Autodesk Inventor part; units mm, degrees
ref_plane "Work Plane1" through (-27.5, -47.498, -12.7) normal (0, 0, 1) x (1, 0, 0)
ref_plane "Work Plane2" through (-27.5, -47.498, -20.1034) normal (0, -1, 0) x (1, 0, 0)
ref_plane "YZ Plane" through (0, 0, 0) normal (1, 0, 0) x (0, 1, 0)
sketch "Sketch1" plane through (0, 0, 0) normal (0, 0, 1) x (1, 0, 0)
  line L0 (4.2148, -12.63) -> (4.2148, -18.63)
  line L1 (0.6968, -12.63) -> (4.2148, -12.63)
  line L2 (0.6968, 12.63) -> (0.6968, -12.63)
  line L3 (16.6988, 12.63) -> (0.6968, 12.63)
  line L4 (16.6988, 17.202) -> (16.6988, 12.63)
  line L5 (21.6388, 17.202) -> (16.6988, 17.202)
  line L6 (21.6388, 12.63) -> (21.6388, 17.202)
  line L7 (23.7568, 12.63) -> (21.6388, 12.63)
  line L8 (23.7568, 18.63) -> (23.7568, 12.63)
  line L9 (-23.7568, 18.63) -> (23.7568, 18.63)
  line L10 (-23.7568, 12.63) -> (-23.7568, 18.63)
  line L11 (-21.6388, 12.63) -> (-23.7568, 12.63)
  line L12 (-21.6388, 17.202) -> (-21.6388, 12.63)
  line L13 (-16.6988, 17.202) -> (-21.6388, 17.202)
  line L14 (-16.6988, 12.63) -> (-16.6988, 17.202)
  line L15 (-0.6968, 12.63) -> (-16.6988, 12.63)
  line L16 (-0.6968, -12.63) -> (-0.6968, 12.63)
  line L17 (-4.2148, -12.63) -> (-0.6968, -12.63)
  line L18 (-4.2148, -18.63) -> (-4.2148, -12.63)
  line L19 (4.2148, -18.63) -> (-4.2148, -18.63)
  line L20 (0, 12.63) -> (10, 12.63)
  line L21 (10, 12.63) -> (-10, 12.63)
  line L22 (10, 12.63) -> (10, -22.37)
  line L23 (10, -22.37) -> (-10, -22.37)
  line L24 (-10, -22.37) -> (-10, 12.63)
  line L25 (-10, 12.63) -> (10, 12.63)
  line L26 (10, 12.63) -> (10, -22.37)
  point P0 (0, 0)
  dimension "d0" = 10
  dimension "d1" = 20
  dimension "d2" = 35
extrude "Extrusion1" add sketch "Sketch1" along normal blind 2 contours L1 L2 L3 L22 L23 L24 L15 L16 L17 L18 L19 L0 | L0 L19 L18 L17 L16 L21 L20 L2 L1
sketch "Sketch2" plane through (0, 0, 0) normal (0, 0, -1) x (-1, 0, 0)
  line L0 (9.2308, -18.63) -> (23.7568, -18.63)
  line L1 (4.2148, -19.63) -> (-4.2148, -19.63)
  line L2 (10, 12.63) -> (10, -22.37)
  line L3 (-10, -22.37) -> (-10, 12.63)
  line L4 (10, -19.63) -> (-10, -19.63)
  line L5 (-10, -19.63) -> (-10, -22.37)
  line L6 (-10, -22.37) -> (10, -22.37)
  line L7 (10, -22.37) -> (10, -19.63)
  point P0 (0, 0)
ref_plane "Work Plane1" through (-27.5, -47.498, -12.7) normal (0, 0, 1) x (1, 0, 0)
extrude "Extrusion2" add sketch "Sketch2" along normal up to surface (12.7 mm away)
sketch "Sketch3" plane through (-10, -22.37, 2) normal (0, -1, 0) x (1, 0, 0)
  line L0 (0, -14.7) -> (0, 0)
  line L1 (0, -14.7) -> (0, -12.7)
  line L2 (20, -14.7) -> (20, 0)
  line L3 (0, -12.7) -> (20, -12.7)
  line L4 (20, -12.7) -> (20, -14.7)
  line L5 (20, -14.7) -> (0, -14.7)
  line L6 (0, -14.7) -> (0, -12.7)
  point P0 (10, -2)
  dimension "d7" = 2
ref_plane "Work Plane2" through (-27.5, -47.498, -20.1034) normal (0, -1, 0) x (1, 0, 0)
extrude "Extrusion3" add sketch "Sketch3" along normal up to surface (25.128 mm away)
properties part number "SyringeConnector"
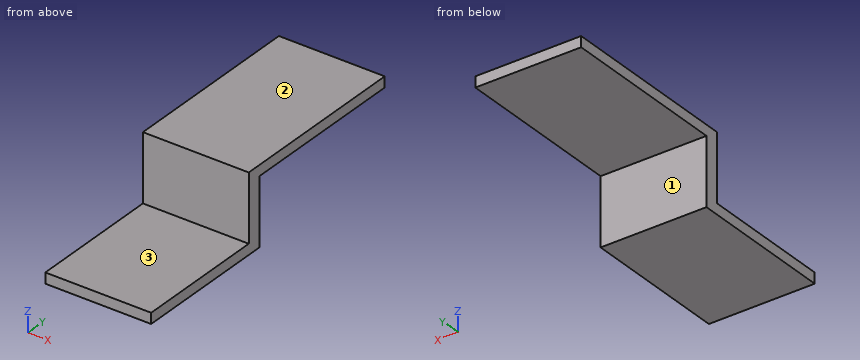
Build history of the part. All positions in model axes, mm. Face numbers are marked on the shaded views. A direction names the side the tool comes from. Coordinates: 2 decimals unless noted, no trailing zeros. Write each loop counter-clockwise with the first axis right and the second up, starting at its lowest first coordinate (ties: lowest second). Pieces come first, ordered by that corner, then holes.
(1) Drill centre lines: line 1 (Y direction, x = 9.25, z = -1.5); line 2 (Z direction, x = -5.75, y = -9.5); line 3 (Z direction, x = -4, y = -30.5). Where is each one in solid material? Low to high.
(2) Cut at C-C on y = -29. List the corners of the cut face in (x, z), and give its area (3 significant figures).
(3) Cut at B-B on z = -2. List the corners of the cut face in (x, y).
(4) 3-axis set-ups, long thin cutter, end or side, ignore diameter. For the marked faces 1, 2 and 3: which of +Z, -Z, +X, -X, +Y, -Y reach the whole face in a straight line?
(5) Cut at A-A on x = -6.5. List the corners of the cut face in (y, z).
(6) Pin check, flat tips, straight feed: pin 1 Ø3 at (x, z) = (-4, -9) entering from +Y; pin 2 Ø10 at (x, y) = (3, -8.5) entering from -Z. Stop position of each tip, or through.
Working result:
1. line 1: y = -22.37 to -19.63
1. line 2: z = 0 to 2
1. line 3: z = -12.7 to -10.7
2. outline: (-10, -12.7) - (10, -12.7) - (10, -10.7) - (-10, -10.7) - close
2. area: 40.0 mm2
3. outline: (-10, -22.37) - (10, -22.37) - (10, -19.63) - (-10, -19.63) - close
4. face 1: -Z, +X, -X, +Y
4. face 2: +Z, +X, -X, +Y, -Y
4. face 3: +Z, +X, -X, -Y
5. outline: (-47.5, -12.7) - (-19.63, -12.7) - (-19.63, 0) - (12.63, 0) - (12.63, 2) - (-22.37, 2) - (-22.37, -10.7) - (-47.5, -10.7) - close
6. pin 1: stops at y = -19.63
6. pin 2: stops at z = 0
